Verification items for the finished model (mm, model axes). Face numbers are marked on the shaded views. A direction names the side the tool comes from. Coordinates: 2 decimals unless noted, no trailing zeros. Loops run counter-clockwise (first coordinate to the right, second up) from the corner with the lowest first, then second, coordinate; pieces in that order, holes last. Notation, with made-up numbers: (29.25, 30.25) - (83.25, 30.25) arc R11 cw to (83.25, 34.25) - close; hole circle Ø4 at (-11, 0). An arc over 180 degrees is marked (long way). Answer as CSV lines item,"result". Start each with the question number.
1. Material ranges on line 1 (Y direction, x = 0.5, z = 1.75); line 2 (Y direction, x = -25, z = 8.25); line 3 (X direction, y = -7, z = 12), recorded low to high. Write a range as [from, to].
2. Release check for a two-part mould opening along X. For the marked faces 4, 5 and 6 record: pulls with the +X half, pulls with the -X half, needs draft (parallel to the pull), parting line crosses it, or undercut.
3. Gauge pin test, flat ends, axial feed: P1, Ø1.5, axis at y = -12.5, z = 11, coming from the -X side; P2, Ø2, axis at x = -35.5, z = 15.5, coming from the -Y side; P3, Ø1.5, axis at x = 12.5, z = 21, coming from the -Y side. Record the tip position at first contact, or that the pin passes through.
4. Set-up check for the marked faces 1, 2 and 3: record each of +Z, -Z, +X, -X, +Y, -Y from which the full face is reachable in a straight line by a thin tool's end or side.
5. Cross-section at A-A (z = 11). Enter the section's corners in (x, y).
```python
from build123d import *

# Parameters (mm, degrees)
F1_DEPTH = 25.4
F2_R     = 4.99999
F3_R     = 4.99999


# Not quite as in the source:
# - a fillet or chamfer is up to 0.001 mm smaller than in the source, because OpenCascade refuses the exact size


with BuildPart() as f1:
    # F0 (on Top) → F1 (new body)
    with BuildSketch(Plane.XY):
        with BuildLine():
            Line((33.5641757438, 33.0211686649), (-50.0175157615, 18.7475354366))
            ThreePointArc((-50.0175157615, 18.7475354366), (-70.4930751684, -8.8439952597), (-43.8361644944, -30.5223303552))
            Line((-43.8361644944, -30.5223303552), (40.6811656436, -23.7064175959))
            ThreePointArc((40.6811656436, -23.7064175959), (66.7727246476, 8.377243564), (33.5641757438, 33.0211686649))
        make_face()
        with BuildLine():
            Line((39.8773238571, -13.7387780367), (-44.640006281, -20.554690796))
            ThreePointArc((-44.640006281, -20.554690796), (-60.5708580224, -7.5991631795), (-48.3341399261, 8.8902413963))
            Line((-48.3341399261, 8.8902413963), (35.2475515791, 23.1638746246))
            ThreePointArc((35.2475515791, 23.1638746246), (56.8505075016, 7.1324114838), (39.8773238571, -13.7387780367))
        make_face(mode=Mode.SUBTRACT)
    extrude(amount=F1_DEPTH)

    # F2 (radius 5 in the source; OpenCascade refuses exactly that, so slightly less here)
    f2_edges = [f1.edges().sort_by_distance(p)[0] for p in [
        (-2.381341, -17.146734, 25.4),
        (-1.577499, -27.114374, 25.4),
    ]]
    fillet(f2_edges, radius=F2_R)

    # F3 (radius 5 in the source; OpenCascade refuses exactly that, so slightly less here)
    f3_edges = [f1.edges().sort_by_distance(p)[0] for p in [
        (-1.577499, -27.114374, 0),
        (66.772725, 8.377244, 0),
        (-8.22667, 25.884352, 0),
        (-70.493075, -8.843995, 0),
        (56.850508, 7.132411, 0),
        (-2.381341, -17.146734, 0),
        (-60.570858, -7.599163, 0),
        (-6.543294, 16.027058, 0),
    ]]
    fillet(f3_edges, radius=F3_R)


solid = f1.part
```
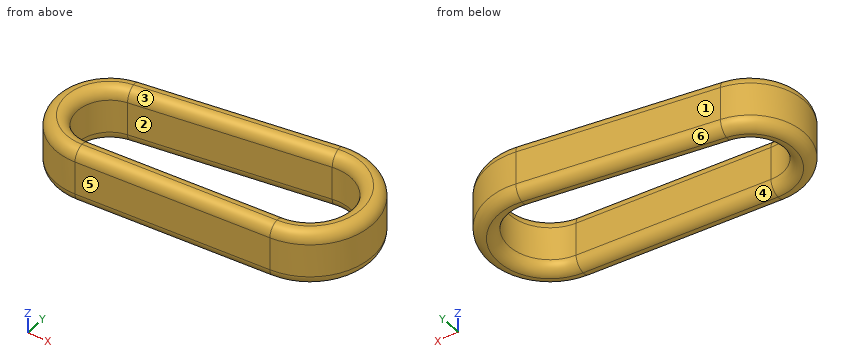
Values follow:
1,line 1,"y = [-25.74, -18.12], [18.45, 26.16]"
1,line 2,"y = [-29, -18.97], [12.88, 23.02]"
1,line 3,"x = [-70.65, -60.63], [52.76, 64.44]"
2,face 4,"undercut"
2,face 5,"pulls with the +X half"
2,face 6,"pulls with the -X half"
3,P1,"stops at x = -69.95"
3,P2,"stops at y = -29.93"
3,P3,"stops at y = -26.03"
4,face 1,"+Z, -Z, -X, +Y"
4,face 2,"+Z, -Z"
4,face 3,"+Z"
5,outline,"(-50.02, 18.75) arc R24.85 ccw to (-43.84, -30.52) - (40.68, -23.71) arc R28.61 ccw (long way) to (33.56, 33.02) - close; hole (-48.33, 8.89) arc R14.85 ccw to (-44.64, -20.55) - (39.88, -13.74) arc R18.61 ccw (long way) to (35.25, 23.16) - close"
